Could you check a few things on this model? Use its own coordinates, in mm. A direction names the side the tool comes from. Coordinates: 2 decimals unless noted, no trailing zeros. Loops run counter-clockwise (first coordinate to the right, second up) from the corner with the lowest first, then second, coordinate; pieces in that order, holes last.
1) If I drill on line 1 along X through (y, z) = (6, 0.9); line 2 along X through (y, z) = (11, 0.6); line 3 along X through (y, z) = (14.5, 1.5), over which ranges is the centre line in solid material (lowest first)?
2) Will these pins go through, and if not, where does the flat tip stop? P1, Ø5, axis at x = 3.19, y = 5.2, coming from the +Z side; P2, Ø1, axis at x = 4.5, z = 0.5, coming from the -Y side.
3) Thinking about a two-plate mould opening in X: for faces 1 (the face through (2.998, 6.683, 1.014)), 2 (the face through (-0.91, 16.3, 1.01)), 3 (the face through (18, 14, 1)), which applies, released by +X, released by -X, zero draft, split by the parting line, or undercut?
4) Imagine slicing it at A-A on z = 0.8. Give the number of separate pieces and of enclosed holes in the cut face, plus the area to 3 significant figures.
5) Imagine slicing it at C-C on x = -12. Please give me the cut outline in (y, z), plus the area to 3 significant figures.
6) For faces 4 (the face through (10.416, 6.014, 0.986)), 5 (the face through (0, 9, 1)), which set-ups out of +Z, -Z, +X, -X, +Y, -Y let a thin tool reach every point of the face, with its end or its side?
7) Imagine slicing it at B-B on y = 27. Please give me the cut outline in (x, z), plus the area to 3 significant figures.
Autodesk Inventor part; units mm, degrees
ref_plane "YZ Plane" through (0, 0, 0) normal (1, 0, 0) x (0, 1, 0)
ref_plane "XZ Plane" through (0, 0, 0) normal (0, 1, 0) x (-1, 0, 0)
ref_plane "XY Plane" through (0, 0, 0) normal (0, 0, 1) x (1, 0, 0)
sketch "Sketch1" plane through (0, 0, 0) normal (0, 0, 1) x (1, 0, 0)
  line L0 (0, 0) -> (18, 0)
  line L1 (18, 0) -> (18, 30)
  line L2 (18, 30) -> (0, 30)
  line L3 (0, 30) -> (0, 0)
  line L4 (0, 0) -> (18, 10.3923)
  line L5 (0, 0) -> (20.7846, 0) construction
  dimension "d0" = 18
  dimension "d1" = 30
  dimension "d2" = 30
extrude "Extrusion1" add sketch "Sketch1" along normal blind 2 contours L3 L2 L1 L4
fillet "Fillet1" radius 3 2 edges at (0, 0, 1) (18, 10.3923, 1)
sketch "Sketch2" plane through (0, 0, 2) normal (0, 0, 1) x (1, 0, 0)
  arc A0 (0, 5.1962) -> (4.5, 2.5981) centre (3, 5.1962) ccw
  arc A1 (16.5, 9.5263) -> (18, 12.1244) centre (15, 12.1244) ccw
  line L0 (4.5, 2.5981) -> (16.5, 9.5263)
  line L1 (10.5, 6.0622) -> (8.7793, 8.5196)
  line L2 (10.5, 6.0622) -> (13.5, 6.0622) construction
  line L3 (8.7793, 8.5196) -> (3.1932, 5.1962)
  line L4 (3.1932, 5.1962) -> (14.3654, 11.8431)
  circle A2 centre (3.1932, 5.1962) radius 1.5
  circle A3 centre (14.3654, 11.8431) radius 1.5
  point P0 (0, 0)
  dimension "d8" = 3
  dimension "d9" = 125
  dimension "d10" = 6.5
  dimension "d11" = 13
  dimension "d12" = 3
  dimension "d13" = 3
extrude "Extrusion2" cut sketch "Sketch2" against normal blind 2
sketch "Sketch3" plane through (0, 0, 2) normal (0, 0, 1) x (1, 0, 0)
  line L0 (18, 12.1244) -> (18, 30)
  line L1 (18, 30) -> (4.0584, 13.3851)
  line L2 (18, 30) -> (39.6893, 30) construction
  line L3 (4.0584, 13.3851) -> (-34.2438, 45.5244)
  line L4 (-34.2438, 45.5244) -> (-20.9174, 62.6556)
  line L5 (-20.9174, 62.6556) -> (18, 30)
  point P0 (0, 0)
  dimension "d16" = 130
  dimension "d17" = 50
  dimension "d18" = 90
extrude "Extrusion3" cut sketch "Sketch3" against normal blind 2
extrude "Extrusion4" add sketch "Sketch3" against normal blind 2
fillet "Fillet2" radius 10 2 edges at (18, 30, 1) (0, 16.7905, 1)
chamfer "Chamfer1" distance 5 distance2 40 1 edges at (-20.9174, 62.6556, 1) measured on face at (-25.3595, 56.9452, 1.3333)
fillet "Fillet3" radius 20 1 edges at (9.7244, 36.9441, 1)
sketch "Sketch4" plane through (0, 0, 2) normal (0, 0, 1) x (1, 0, 0)
  line L0 (-23.9874, 58.7091) -> (8.6742, 37.6221)
  line L1 (-7.6566, 48.1656) -> (18, 18.7306)
  line L2 (18, 12.1244) -> (18, 25.3369)
  line L3 (-7.6566, 48.1656) -> (3.9893, 54.5621)
  line L4 (3.9893, 54.5621) -> (27.8287, 24.1291)
  line L5 (27.8287, 24.1291) -> (18, 18.7306)
  point P0 (0, 0)
extrude "Extrusion5" cut sketch "Sketch4" against normal blind 2
fillet "Fillet4" radius 5 1 edges at (18, 18.7306, 1)
sketch "Sketch5" plane through (0, 0, 2) normal (0, 0, 1) x (1, 0, 0)
  line L0 (16.7692, 20.1427) -> (-7.6566, 48.1656)
  line L1 (0, 39.3814) -> (-29.1156, 52.1168)
  line L2 (-34.2438, 45.5244) -> (-23.9874, 58.7091)
  line L3 (-29.1156, 52.1168) -> (-28.0652, 63.5725)
  line L4 (-28.0652, 63.5725) -> (-0.6496, 57.8446)
  line L5 (-0.6496, 57.8446) -> (0, 39.3814)
  point P0 (0, 0)
extrude "Extrusion6" cut sketch "Sketch5" against normal blind 2
fillet "Fillet5" radius 20 1 edges at (0, 39.3814, 1)
fillet "Fillet6" radius 3 1 edges at (-29.1156, 52.1168, 1)
chamfer "Chamfer2" distance 20 distance2 3 1 edges at (-34.2438, 45.5244, 1) measured on face at (-24.0199, 36.9456, 1.3333)
fillet "Fillet7" radius 2 1 edges at (-32.4018, 47.8923, 1)
sketch "Sketch6" plane through (0, 0, 2) normal (0, 0, 1) x (1, 0, 0)
  line L0 (-31.3011, 46.6491) -> (-18.9229, 32.6687)
  arc A0 (0, 12.1274) -> (-3.5721, 19.7878) centre (-10, 12.1274) ccw
  line L1 (-31.3011, 46.6491) -> (-3.5721, 19.7878)
  line L2 (-3.5721, 19.7878) -> (-20.8807, 12.1274)
  arc A1 (-31.3823, 49.203) -> (-31.3011, 46.6491) centre (-29.8037, 47.9749) ccw
  line L3 (-20.8807, 12.1274) -> (-31.3011, 46.6491)
  point P0 (0, 0)
extrude "Extrusion7" cut sketch "Sketch6" against normal blind 10
properties part number "Claw Tip"
Filled in:
1. line 1: x = 0 to 1.93, 4.46 to 10.39
1. line 2: x = 0 to 13.12, 15.61 to 17.78
1. line 3: x = -0.29 to 18
2. P1: stops at z = 2
2. P2: stops at y = 2.37
3. face 1: undercut
3. face 2: released by -X
3. face 3: released by +X
4. separate pieces: 1
4. enclosed holes: 2
4. area: 866 mm2
5. outline: (27.95, 0) - (44.63, 0) - (44.63, 2) - (27.95, 2) - close
5. area: 33.4 mm2
6. face 4: +Z, -Z, +X, -Y
6. face 5: +Z, -Z, -X, -Y
7. outline: (-11.02, 0) - (10.79, 0) - (10.79, 2) - (-11.02, 2) - close
7. area: 43.6 mm2
